from build123d import *

# Parameters (mm, degrees)
PAD_DEPTH       = 5
SKETCH001_R     = 6
SKETCH001_R_2   = 3.8
POCKET_DEPTH    = 0.8
SKETCH004_W     = 19.5
SKETCH004_H     = 3
POCKET001_DEPTH = 5
SKETCH011_R     = 1.75
POCKET002_DEPTH = 5
FILLET_R        = 3


with BuildPart() as part:
    # Sketch → Pad (new body)
    with BuildSketch(Plane.XY):
        Polygon((-21, 22), (21, 22), (12.5, -12.5), (-12.5, -12.5), align=None)
    extrude(amount=PAD_DEPTH)

    # Sketch001 → Pocket (cut)
    with BuildSketch(Plane(origin=(0, 0, 0), x_dir=(1, 0, 0), z_dir=(0, 0, -1))):
        Circle(SKETCH001_R)
        Circle(SKETCH001_R_2, mode=Mode.SUBTRACT)
    extrude(amount=-POCKET_DEPTH, mode=Mode.SUBTRACT)

    # Sketch004 → Pocket001 (cut)
    with BuildSketch(Plane.XY.offset(5)):
        with Locations((0, 9.5)):
            Rectangle(SKETCH004_W, SKETCH004_H)
    extrude(amount=-POCKET001_DEPTH, mode=Mode.SUBTRACT)

    # Sketch011 → Pocket002 (cut)
    with BuildSketch(Plane(origin=(0, 0, 0), x_dir=(1, 0, 0), z_dir=(0, 0, -1))):
        with Locations((-8, 8)):
            Circle(SKETCH011_R)
        with Locations((8, 8)):
            Circle(SKETCH011_R)
        with Locations((-14, -12)):
            Circle(SKETCH011_R)
        with Locations((14, -12)):
            Circle(SKETCH011_R)
    extrude(amount=-POCKET002_DEPTH, mode=Mode.SUBTRACT)

    # Fillet
    fillet_edges = [part.edges().sort_by_distance(p)[0] for p in [
        (21, 22, 2.5),
        (-21, 22, 2.5),
        (-12.5, -12.5, 2.5),
        (12.5, -12.5, 2.5),
    ]]
    fillet(fillet_edges, radius=FILLET_R)


solid = part.part
Work out the finished part from the listing and answer in its coordinate system (mm). A direction names the side the tool comes from. Round coordinates to 2 decimals unless told otherwise and drop trailing zeros. Order: outer loops, then holes, each group sorted by start corner. A loop starts at its lowest first (then second) coordinate and runs counter-clockwise, first axis right, second up. Notation, with made-up numbers: M 50,28.25 L 107,28.25 A14 ccw 107,54.25 Z; hole C -38.75,-5.5 d11. An arc over 180 degrees is marked long. Put each result on its own line as item: value. Start each with the question number.
Q1. Section C-C, the plane z = 3.05 is taken. Write down the section's boundary in (x, y).
Q2. Section D-D, the plane x = 15 is taken. Write down the section's boundary in (y, z), and give its area (3 significant figures).
Q3. Section B-B, the plane y = 9.5 is taken. Write down the section's boundary in (x, z).
Q4. For a pull along X with two mould halves and no side action, classify faces 1 (the flat face through (16.62, 4.23, 2.46)), 2 (the flat face through (0, 5, 5)), 3 (the cylindrical face through (-6.331, -8.526, 2.465)), 4 (the flat face through (-16.524, 3.833, 2.465)) as pulls with the +X half, pulls with the -X half, needs draft (parallel to the pull), parting line crosses it, or undercut.
Q5. Flat-ended cylindrical pins translate along their axes: pin 1 (3 mm diameter, centred on y = 0, z = 4, fed in from +X); pin 2 (1.5 mm diameter, centred on y = 9, z = 2.5, fed in from -X); pin 3 (1.5 mm diameter, centred on y = 9, z = 3.5, fed in from +X). Find the tip coordinate at first contact, or state that the pin passes through.
Q6. Section A-A, the plane x = -8 is taken. Write down the section's boundary in (y, z).
Q7. Straight lines are drawn through the part: L1, parallel to Y at x = -8, z = 3.4; L2, parallel to Y at x = 0, z = 0.65; L3, parallel to X at y = -8, z = 3.65. For each, find the intervals that lie inside material, in ascending order. Write a range as [from, to].
Q8. A tool of negligible diameter and unlimited length cuts with its end or side. For faces 5 (the cylindrical face through (-3.796, -0.167, 0.394)), 6 (the flat face through (0, 8, 3)), 7 (the flat face through (0, -12.5, 2)), from which of +Z, -Z, +X, -X, +Y, -Y can it reach the whole face along a straight path? Write none if from no direction.
Findings below:
1. outline: M -20.08,18.28 L -13.06,-10.22 A3 ccw -10.15,-12.5 L 10.15,-12.5 A3 ccw 13.06,-10.22 L 20.08,18.28 A3 ccw 17.17,22 L -17.17,22 A3 ccw Z; hole C -14,12 d3.5; hole C -8,-8 d3.5; hole M -9.75,8 L 9.75,8 L 9.75,11 L -9.75,11 Z; hole C 8,-8 d3.5; hole C 14,12 d3.5
2. outline: M -2.35,0 L 10.56,0 L 10.56,5 L -2.35,5 Z; M 13.44,0 L 22,0 L 22,5 L 13.44,5 Z
2. area: 107 mm^2
3. outline: M -17.92,0 L -9.75,0 L -9.75,5 L -17.92,5 Z; M 9.75,0 L 17.92,0 L 17.92,5 L 9.75,5 Z
4. face 1: pulls with the +X half
4. face 2: needs draft
4. face 3: undercut
4. face 4: pulls with the -X half
5. pin 1: stops at x = 15.95
5. pin 2: stops at x = -17.98
5. pin 3: stops at x = 17.98
6. outline: M -12.5,0 L -9.75,0 L -9.75,5 L -12.5,5 Z; M -6.25,0 L 8,0 L 8,5 L -6.25,5 Z; M 11,0 L 22,0 L 22,5 L 11,5 Z
7. L1: y = [-12.5, -9.75], [-6.25, 8], [11, 22]
7. L2: y = [-12.5, -6], [-3.8, 3.8], [6, 8], [11, 22]
7. L3: x = [-13.61, -9.75], [-6.25, 6.25], [9.75, 13.61]
8. face 5: -Z
8. face 6: +Z, -Z
8. face 7: +Z, -Z, +X, -X, -Y
